Study the drawing (mm; zero at the part's minimum x, y, z) and answer. A direction names the side the tool comes from. Give positions to 0.01 mm unless a question says otherwise; leave off trailing zeros. Order: outer loops, then holes, each group sorted by start corner. A loop starts at its lowest first (then second) coordinate and runs counter-clockwise, first axis right, second up. Notation, with made-up numbers: (-2.5, 13.5) - (52.5, 13.5) arc R21 cw to (52.5, 34.5) - close; hole circle Ø5 at (24, 4). An arc over 180 degrees is marked (long way). Return JSON: item names as keys, results as strings.
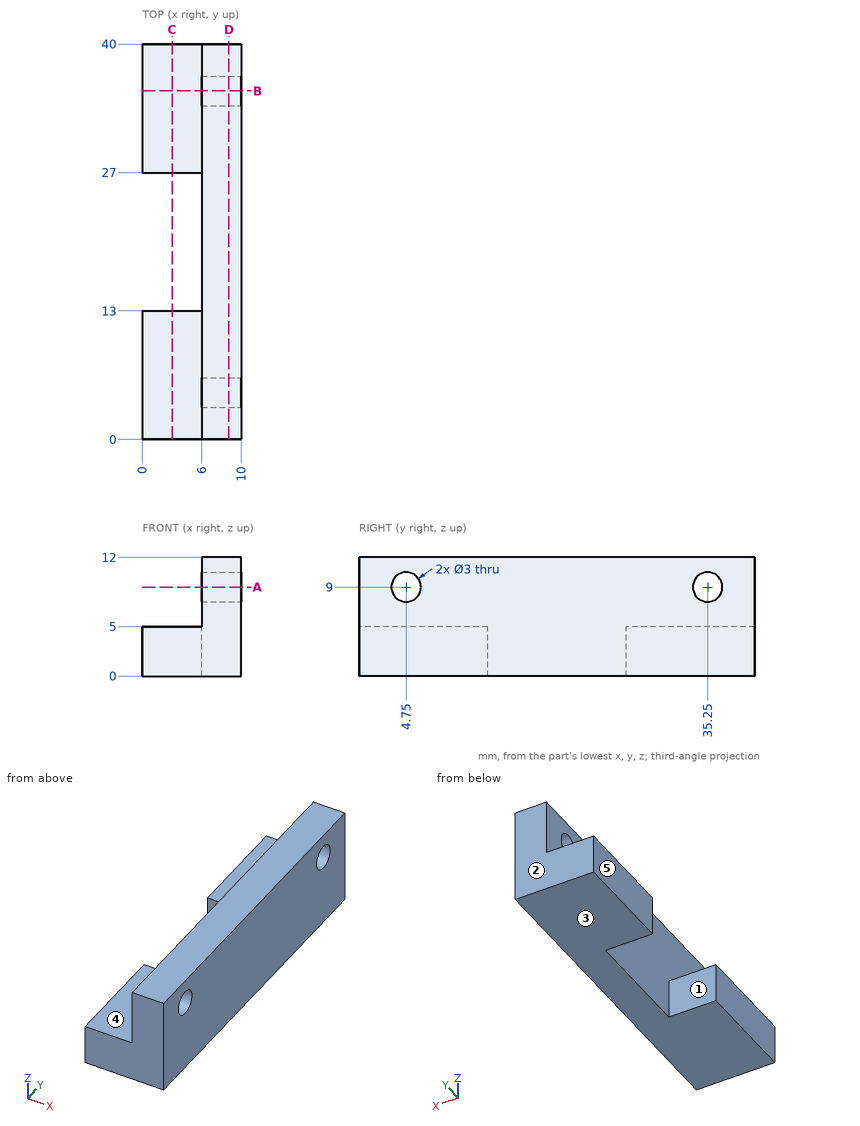
Q1. A cutting plane is placed at B-B (y = 35.25). Write down the section's boundary in (x, z).
Values:
{"outline": "(0, 0) - (10, 0) - (10, 7.5) - (6, 7.5) - (6, 5) - (0, 5) - close; (6, 10.5) - (10, 10.5) - (10, 12) - (6, 12) - close"}
Q2. Determine the mould class of the marked faces 1, 2 and 3 for opening direction Y: released by +Y, released by -Y, zero draft, split by the parting line, or undercut.
Values:
{"face 1": "undercut", "face 2": "released by +Y", "face 3": "zero draft"}
Q3. A cutting plane is placed at D-D (x = 8.75). Write down the section's boundary in (y, z).
Values:
{"outline": "(0, 0) - (40, 0) - (40, 12) - (0, 12) - close; hole circle Ø3 at (4.75, 9); hole circle Ø3 at (35.25, 9)"}
Q4. Consider L1, parallel to Z at x = 8.4, y = 4.75; L2, parallel to Z at x = 4, y = 11.5; L3, parallel to Y at x = 1, z = 1. Determine where each line is inside the solid, lowest interval first.
Values:
{"L1": "z = 0 to 7.5, 10.5 to 12", "L2": "z = 0 to 5", "L3": "y = 0 to 13, 27 to 40"}
Q5. A cutting plane is placed at C-C (x = 3). Write down the section's boundary in (y, z).
Values:
{"outline": "(0, 0) - (13, 0) - (13, 5) - (0, 5) - close; (27, 0) - (40, 0) - (40, 5) - (27, 5) - close"}
Q6. Given pin 1 (3 mm diameter, centred on x = 2, y = 32.5, fed in from +Z); pin 2 (6 mm diameter, centred on y = 18, z = 7, fed in from -X); pin 3 (1.8 mm diameter, centred on y = 4.75, z = 9, fed in from +X), each flat-ended and moving along its own axis, determine where each tip first touches the part or whether it passes through.
Values:
{"pin 1": "stops at z = 5", "pin 2": "stops at x = 6", "pin 3": "passes through"}
Q7. A cutting plane is placed at A-A (z = 9). Write down the section's boundary in (x, y), and give its area (3 significant figures).
Values:
{"outline": "(6, 0) - (10, 0) - (10, 3.25) - (6, 3.25) - close; (6, 6.25) - (10, 6.25) - (10, 33.75) - (6, 33.75) - close; (6, 36.75) - (10, 36.75) - (10, 40) - (6, 40) - close", "area": "136 mm²"}
Q8. For the marked faces 4 and 5, determine the directions among +Z, -Z, +X, -X, +Y, -Y from which every point of the face is accessible in a straight line to the end or side of a thin tool.
Values:
{"face 4": "+Z, -X, +Y, -Y", "face 5": "+Z, -Z, -X, +Y, -Y"}
